Check sheet for the modelled part. Datum: model origin and axes. Units: mm. Round coordinates to 2 decimals unless told otherwise and drop trailing zeros. Write each loop counter-clockwise with the first axis right and the second up, starting at its lowest first coordinate (ties: lowest second). Pieces come first, ordered by that corner, then holes. Notation, with made-up numbers: (-12, 31.5) -> (4, 31.5) arc R14 cw to (4, 38.5) -> close; hole circle Ø11 at (-5, 43). An arc over 180 degrees is marked (long way). Answer as a JSON object with one key per item and string values. Group by question number.
```python
from build123d import *

# Parameters (mm, degrees)
SKETCH_R  = 6.25
PAD_DEPTH = 4


with BuildPart() as part:
    # Sketch → Pad (new body)
    with BuildSketch(Plane.XY):
        with BuildLine():
            ThreePointArc((-93.224272, 37.433574), (-111.583346, 29.327163), (-107.580303, 9.661326))
            Line((-107.580303, 9.661326), (-11.350303, -70.098674))
            ThreePointArc((-11.350303, -70.098674), (6.022276, -72.087404), (14.840368, -56.987643))
            Line((11.985276, 0.594268), (14.840368, -56.987643))
            ThreePointArc((11.985276, 0.594268), (9.337508, 7.537304), (3.109296, 11.59018))
            Line((-93.224272, 37.433574), (3.109296, 11.59018))
        make_face()
        Circle(SKETCH_R, mode=Mode.SUBTRACT)
    extrude(amount=PAD_DEPTH)


solid = part.part
```
(1) Scan lines: line 1 along Y through (x, z) = (0, 0.95); line 2 along Y through (x, z) = (-1, 3.25); line 3 along X through (y, z) = (-30, 1.5). Record each from-to range of solid material in increasing order.
(2) Go/stop test with flat-tipped pins: pin 1 Ø1.5 at (x, z) = (-85.5, 1.5) entering from -Y; pin 2 Ø1.5 at (y, z) = (-43, 2) entering from +X; pin 3 Ø2 at (x, z) = (-77.5, 3) entering from +Y; pin 4 Ø8 at (x, y) = (-66.5, -31.5) entering from +Z. Record where each tip stops, or that it passes through.
(3) Section check A-A on z = 3.4. Record the cut outline in (x, y).
(4) Section check C-C on y = -36.5. Record the cut outline in (x, z).
(5) Release check for a two-part mould opening along Y. For faces 1 (the cylindrical face through (5.96, 1.88, 1.97)), 2 (the flat face through (-45.732, 24.693, 1.972)), 3 (the flat face through (-60.14, -29.66, 1.97)) record: pulls with the +Y half, pulls with the -Y half, needs draft (parallel to the pull), parting line crosses it, or undercut.
(6) Section check B-B on x = 0. Record the cut outline in (y, z).
(7) Section check D-D on x = -71. Record the cut outline in (y, z).
Data:
{
 "1": {"line 1": "y = -73.74 to -6.25, 6.25 to 12.42", "line 2": "y = -73.78 to -6.17, 6.17 to 12.69", "line 3": "x = -59.73 to 13.5"},
 "2": {"pin 1": "stops at y = -9.26", "pin 2": "stops at x = 14.18", "pin 3": "stops at y = 33.48", "pin 4": "passes through"},
 "3": {"outline": "(-107.58, 9.66) -> (-11.35, -70.1) arc R16 ccw to (14.84, -56.99) -> (11.99, 0.59) arc R12 ccw to (3.11, 11.59) -> (-93.22, 37.43) arc R16 ccw to start; hole circle Ø12.5 at (0, 0)"},
 "4": {"outline": "(-51.89, 0) -> (13.82, 0) -> (13.82, 4) -> (-51.89, 4) -> close"},
 "5": {"face 1": "undercut", "face 2": "pulls with the +Y half", "face 3": "pulls with the -Y half"},
 "6": {"outline": "(-73.74, 0) -> (-6.25, 0) -> (-6.25, 4) -> (-73.74, 4) -> close; (6.25, 0) -> (12.42, 0) -> (12.42, 4) -> (6.25, 4) -> close"},
 "7": {"outline": "(-20.66, 0) -> (31.47, 0) -> (31.47, 4) -> (-20.66, 4) -> close"}
}
